CAD build for the part. Positions are in the model's coordinates, mm. Face numbers are marked on the shaded views. Round coordinates to 2 decimals unless told otherwise and drop trailing zeros. Loops run counter-clockwise (first coordinate to the right, second up) from the corner with the lowest first, then second, coordinate; pieces in that order, holes last.
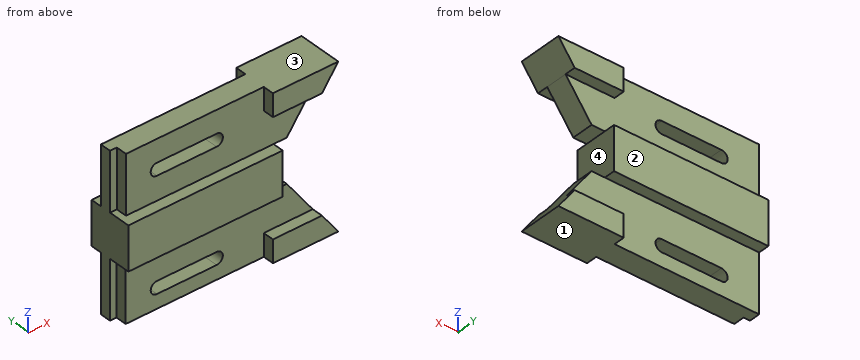
from build123d import *

# Parameters (mm, degrees)
F1_DEPTH = 12.7
F2_DEPTH = 6.35
F3_DEPTH = 12.7
F0_W     = 3.919005394
F0_H     = 33.7724040388
F0_W_2   = 3.7486106157
F4_DEPTH = 6.35


with BuildPart() as f1:
    # F0 (on Front) → F1 (new body, symmetric)
    with BuildSketch(Plane.XZ):
        Polygon((-63.2172524929, 25.2362620085), (-67.1362578869, 25.2362620085), (-67.1362578869, 12.6181310043), (22.1488550305, 12.6181310043), (22.1488550305, 25.2362620085), align=None)
        Polygon((22.1488550305, 12.6181310043), (-67.1362578869, 12.6181310043), (-67.1362578869, 0), (-63.3876472712, 0), (22.1488550305, 0), align=None)
    extrude(amount=F1_DEPTH, both=True)

    # F0 (on Front) → F2 (join, symmetric)
    with BuildSketch(Plane.XZ):
        Polygon((16.5259391069, 59.0086660474), (-63.2172524929, 59.0086660474), (-63.2172524929, 25.2362620085), (22.1488550305, 25.2362620085), (29.8164691776, 25.2362620085), (44.8951655051, 45.9909210103), (16.5259391069, 45.9909210103), align=None)
        with BuildLine():
            ThreePointArc((-45.3261546791, 38.8342062133), (-48.9041308958, 42.4647925685), (-45.2217078929, 45.9893963645))
            Line((-45.2217078929, 45.9893963645), (-10.7368518343, 45.9909210068))
            ThreePointArc((-10.7368518343, 45.9909210068), (-7.1583362305, 42.4126427149), (-10.7366936281, 38.8342062133))
            Line((-10.7366936281, 38.8342062133), (-45.3261546791, 38.8342062133))
        make_face(mode=Mode.SUBTRACT)
        Polygon((29.8164691776, 0), (22.1488550305, 0), (-63.3876472712, 0), (-63.3876472712, -33.7724040388), (16.5259391069, -33.7724040388), (16.5259391069, -20.7546590018), (44.8951655051, -20.7546590018), align=None)
        with BuildLine():
            ThreePointArc((-45.3399057596, -25.7136520276), (-48.9045054721, -22.1284454979), (-45.3261546791, -18.5569636524))
            Line((-45.3261546791, -18.5569636524), (-10.7366936281, -18.5569636524))
            ThreePointArc((-10.7366936281, -18.5569636524), (-7.1583362296, -22.135322417), (-10.7366963604, -25.7136784494))
            Line((-10.7366963604, -25.7136784494), (-45.3124090631, -25.7136520486))
            ThreePointArc((-45.3124090631, -25.7136520486), (-45.3261574114, -25.7136784494), (-45.3399057596, -25.7136520276))
        make_face(mode=Mode.SUBTRACT)
    extrude(amount=F2_DEPTH, both=True)

    # F0 (on Front) → F3 (join, symmetric)
    with BuildSketch(Plane.XZ):
        Polygon((54.3528310955, 59.0086660474), (16.5259391069, 59.0086660474), (16.5259391069, 45.9909210103), (44.8951655051, 45.9909210103), align=None)
        Polygon((54.3528310955, -33.7724040388), (44.8951655051, -20.7546590018), (16.5259391069, -20.7546590018), (16.5259391069, -33.7724040388), align=None)
    extrude(amount=F3_DEPTH, both=True)

    # F0 (on Front) → F4 (join)
    with BuildSketch(Plane.XZ):
        with Locations((-65.1767551899, 42.122464028)):
            Rectangle(F0_W, F0_H)
        with Locations((-65.261952579, -16.8862020194)):
            Rectangle(F0_W_2, F0_H)
    extrude(amount=-F4_DEPTH)


solid = f1.part
Item 1: Mould opens along Z. For the marked faces 1, 2, 3 and 4 say: released by +Z, released by -Z, zero draft, split by the parting line, or undercut.
Verdict:
face 1: released by -Z
face 2: zero draft
face 3: released by +Z
face 4: undercut
Item 2: Cut at B-B (y = 1.5). State how many separate pieces and enclosed holes the cut face has, plus the area to 4 significant figures.
Verdict:
separate pieces: 1
enclosed holes: 2
area: 9,055 mm2
Item 3: Cut at A-A (y = -10.5). List the corners of the cut face in (x, z).
Verdict:
outline: (-67.14, 0) - (22.15, 0) - (22.15, 25.24) - (-67.14, 25.24) - close; (16.53, -33.77) - (54.35, -33.77) - (44.9, -20.75) - (16.53, -20.75) - close; (16.53, 45.99) - (44.9, 45.99) - (54.35, 59.01) - (16.53, 59.01) - close
Item 4: Cut at C-C (x = -14). List the corners of the cut face in (y, z), plus the area to 3 significant figures.
Verdict:
outline: (-12.7, 0) - (-6.35, 0) - (-6.35, -18.56) - (6.35, -18.56) - (6.35, 0) - (12.7, 0) - (12.7, 25.24) - (6.35, 25.24) - (6.35, 38.83) - (-6.35, 38.83) - (-6.35, 25.24) - (-12.7, 25.24) - close; (-6.35, -33.77) - (6.35, -33.77) - (6.35, -25.71) - (-6.35, -25.71) - close; (-6.35, 45.99) - (6.35, 45.99) - (6.35, 59.01) - (-6.35, 59.01) - close
area: 1,320 mm2
Item 5: Cut at D-D (x = 32.5). List the corners of the cut face in (y, z), plus the area to 3 significant figures.
Verdict:
outline: (-12.7, -33.77) - (12.7, -33.77) - (12.7, -20.75) - (6.35, -20.75) - (6.35, -3.69) - (-6.35, -3.69) - (-6.35, -20.75) - (-12.7, -20.75) - close; (-12.7, 45.99) - (-6.35, 45.99) - (-6.35, 28.93) - (6.35, 28.93) - (6.35, 45.99) - (12.7, 45.99) - (12.7, 59.01) - (-12.7, 59.01) - close
area: 1,090 mm2
Item 6: Flat gauge pins, fed straight in: P1, Ø3, axis at y = 9.5, z = 54, coming from the -X side; P2, Ø3, axis at x = -66, z = 49.5, coming from the -Y side; P3, Ø8, axis at x = -41.5, z = -12, coming from the -Y side. Where does each tip first touch, or does it go through?
Verdict:
P1: stops at x = 16.53
P2: stops at y = 0
P3: stops at y = -6.35
Item 7: Wall check: L1, parallel to Z at x = -13.5, y = -3.5; L2, parallel to Z at x = 22.5, y = -1; L3, parallel to Z at x = 32, y = 9.25. Give the ranges that are in metal, low to high.
Verdict:
L1: z = -33.77 to -25.71, -18.56 to 38.83, 45.99 to 59.01
L2: z = -33.77 to 0, 25.24 to 59.01
L3: z = -33.77 to -20.75, 45.99 to 59.01
